Can you work these out from the model? Positions are in its coordinate system, mm. Face numbers are marked on the shaded views. A direction names the side the tool comes from. Give positions to 0.01 mm unless a question says otherwise; leave off trailing zeros. Loops run counter-clockwise (first coordinate to the right, second up) from the corner with the lowest first, then second, coordinate; pieces in that order, holes last. Notation, with made-up numbers: (7.25, 22) - (18.25, 22) arc R12 ccw to (18.25, 42) - close; hole circle Ø1 at (6, -1.5). An arc over 180 degrees is marked (long way). Answer as a JSON object with one key per item and string values.
```python
from build123d import *

# Parameters (mm, degrees)
F0_R          = 6.35
F1_DEPTH      = 50.8
F2_R          = 6.708201
F3_DEPTH      = 25.4
F3_DEPTH_BACK = 25.4


with BuildPart() as f1:
    # F0 (on Front) → F1 (new body)
    with BuildSketch(Plane.XZ):
        Circle(F0_R)
    extrude(amount=F1_DEPTH)

    # F2 (on Right) → F3 (join, two sides)
    with BuildSketch(Plane.YZ) as f3_sk:
        with Locations((-8.772769, 0)):
            Circle(F2_R)
    extrude(amount=F3_DEPTH)
    extrude(f3_sk.sketch, amount=-F3_DEPTH_BACK)


solid = f1.part
```
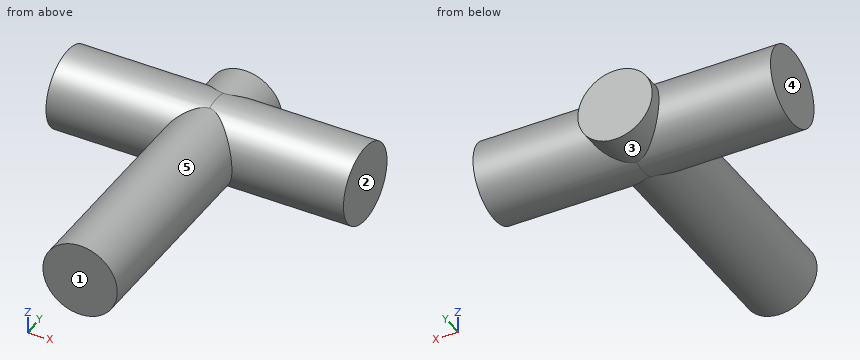
1) Imagine slicing it at B-B on y = -45. Write out the boundary of the cut face in (x, z), and give its area (3 significant figures).
Check sheet entries:
{"outline": "circle Ø12.7 at (0, 0)", "area": "127 mm2"}
2) Imagine slicing it at D-D on z = 3. Write out the boundary of the cut face in (x, y), and give its area (3 significant figures).
Check sheet entries:
{"outline": "(-25.4, -14.77) - (-5.6, -14.77) - (-5.6, -50.8) - (5.6, -50.8) - (5.6, -14.77) - (25.4, -14.77) - (25.4, -2.77) - (5.6, -2.77) - (5.6, 0) - (-5.6, 0) - (-5.6, -2.77) - (-25.4, -2.77) - close", "area": "1,040 mm2"}
3) I'm going to push flat-ended pins straight in: P1, Ø4, axis at x = 4.5, y = -43.5, coming from the +Z side; P2, Ø12, axis at x = -7, y = -43, coming from the +Z side; P3, Ø8, axis at x = -14, z = -1.5, coming from the -Y side. Where does each tip first touch, or does it pass through?
Check sheet entries:
{"P1": "z = 5.84", "P2": "z = 6.27", "P3": "y = -15.48"}
4) Imagine slicing it at A-A on z = 0. Write out the boundary of the cut face in (x, y).
Check sheet entries:
{"outline": "(-25.4, -15.48) - (-6.35, -15.48) - (-6.35, -50.8) - (6.35, -50.8) - (6.35, -15.48) - (25.4, -15.48) - (25.4, -2.06) - (6.35, -2.06) - (6.35, 0) - (-6.35, 0) - (-6.35, -2.06) - (-25.4, -2.06) - close"}
5) I need wall thicknesses on L1, parallel to X at y = -23, z = 4; L2, parallel to X at y = -14.5, z = 4.5; L3, parallel to Y at x = -8, z = -1. Which ranges of each line are inside material? Lowest first, please.
Check sheet entries:
{"L1": "-4.93 to 4.93", "L2": "-4.48 to 4.48", "L3": "-15.41 to -2.14"}
6) Which directions (+Z, -Z, +X, -X, +Y, -Y) give clear straight access to the entire face, cutting with the end or side of a thin tool? Please do the marked faces 4 and 5.
Check sheet entries:
{"face 4": "+Z, -Z, -X, +Y, -Y", "face 5": "-Y"}
7) Imagine slicing it at C-C on x = -3. Write out the boundary of the cut face in (y, z), and give its area (3 significant figures).
Check sheet entries:
{"outline": "(-50.8, -5.6) - (-12.47, -5.6) arc R6.71 ccw to (-5.07, -5.6) - (0, -5.6) - (0, 5.6) - (-5.07, 5.6) arc R6.71 ccw to (-12.47, 5.6) - (-50.8, 5.6) - close", "area": "580 mm2"}
8) If we mould it in two halves opening along X, with no side actions, what happens to the marked faces 1, 2 and 3? For each: released by +X, released by -X, zero draft, split by the parting line, or undercut.
Check sheet entries:
{"face 1": "zero draft", "face 2": "released by +X", "face 3": "split by the parting line"}
